Input: part model. Units: mm. Frame: model coordinates. A direction names the side the tool comes from. Round coordinates to 2 decimals unless told otherwise and drop trailing zeros. Loops run counter-clockwise (first coordinate to the right, second up) from the corner with the lowest first, then second, coordinate; pieces in that order, holes last.
(1) Access query for faces 1 (the face through (13, -732, 55)), 2 (the face through (7, -731, -62.5)). Directions: +Z, -Z, +X, -X, +Y, -Y. A direction counts if a zero-diameter tool reaches every point of the face in a straight line with its end or side. Return the directions, or none.
(2) First-contact query: pin 1 Ø3 at (y, z) = (-462.5, -25.5) entering from +X; pin 2 Ø7.5 at (y, z) = (-1442.5, -58.5) entering from -X. Flat tips, straight axial feed; report the tip coordinate or a pass-through.
(3) Cut plane B-B, the plane y = -822.5. Output: boundary loops of the cut face in (x, z).
(4) Cut plane A-A, the plane x = 11. Output: boundary loops of the cut face in (y, z).
(5) Line query: line 1 (Z direction, x = 9.5, y = -562); line 2 (Z direction, x = -14, y = -471); line 3 (X direction, y = -788, z = 49). Output: solid intervals per line, ascending.
(6) Cut plane C-C, the plane z = 23.5. Output: boundary loops of the cut face in (x, y), and give its area (3 significant figures).
(7) Draft query along Z for faces 3 (the face through (-22, -65, 23)), 4 (the face through (14, -731, -55)), 5 (the face through (8, -732, 62.5)). Return one class per face: released by +Z, released by -Z, zero draft, split by the parting line, or undercut.
from build123d import *

# Parameters (mm, degrees)
F1_DEPTH = 1482.5
F3_DEPTH = 125.001
F5_DEPTH = 10


with BuildPart() as f1:
    # F0 (on Front) → F1 (new body)
    with BuildSketch(Plane.XZ):
        with BuildLine():
            Line((-25.16784, 62.5), (-25.16784, -62.5))
            Line((-25.16784, -62.5), (39.83216, -62.5))
            Line((39.83216, -62.5), (39.83216, -55))
            Line((39.83216, -55), (-12.46784, -55))
            ThreePointArc((-12.46784, -55), (-18.124695, -52.656854), (-20.46784, -47))
            Line((-20.46784, -47), (-20.46784, 47))
            ThreePointArc((-20.46784, 47), (-18.124695, 52.656854), (-12.46784, 55))
            Line((-12.46784, 55), (39.83216, 55))
            Line((39.83216, 55), (39.83216, 62.5))
            Line((39.83216, 62.5), (-25.16784, 62.5))
        make_face()
    extrude(amount=F1_DEPTH)

    # F2 (on face) → F3 (cut, through all)
    with BuildSketch(Plane.XY.offset(62.5)):
        with BuildLine():
            Line((39.83216, 0), (-25.16784, 0))
            Line((-25.16784, 0), (-25.16784, -65))
            Line((-25.16784, -65), (-17.66784, -65))
            Line((-17.66784, -65), (-17.66784, -12.7))
            ThreePointArc((-17.66784, -12.7), (-15.324695, -7.043146), (-9.66784, -4.7))
            Line((-9.66784, -4.7), (39.83216, -4.7))
            Line((39.83216, -4.7), (39.83216, 0))
        make_face()
        with BuildLine():
            Line((-17.66784, -1417.5), (-25.16784, -1417.5))
            Line((-25.16784, -1417.5), (-25.16784, -1482.5))
            Line((-25.16784, -1482.5), (39.83216, -1482.5))
            Line((39.83216, -1482.5), (39.83216, -1477.8))
            Line((39.83216, -1477.8), (-9.66784, -1477.8))
            ThreePointArc((-9.66784, -1477.8), (-15.324695, -1475.456854), (-17.66784, -1469.8))
            Line((-17.66784, -1469.8), (-17.66784, -1417.5))
        make_face()
    extrude(amount=-F3_DEPTH, mode=Mode.SUBTRACT)

    # F4 (on face) → F5 (cut)
    with BuildSketch(Plane.XY.offset(62.5)):
        with BuildLine():
            Line((-17.66784, -65), (39.83216, -65))
            Line((39.83216, -65), (39.83216, -4.7))
            Line((39.83216, -4.7), (-9.66784, -4.7))
            ThreePointArc((-9.66784, -4.7), (-15.324695, -7.043146), (-17.66784, -12.7))
            Line((-17.66784, -12.7), (-17.66784, -65))
        make_face()
        with BuildLine():
            Line((39.83216, -1417.5), (-17.66784, -1417.5))
            Line((-17.66784, -1417.5), (-17.66784, -1469.8))
            ThreePointArc((-17.66784, -1469.8), (-15.324695, -1475.456854), (-9.66784, -1477.8))
            Line((-9.66784, -1477.8), (39.83216, -1477.8))
            Line((39.83216, -1477.8), (39.83216, -1417.5))
        make_face()
    extrude(amount=-F5_DEPTH, mode=Mode.SUBTRACT)


solid = f1.part
Reported:
1. face 1: +X, +Y, -Y
1. face 2: -Z, +X, -X, +Y, -Y
2. pin 1: stops at x = -20.47
2. pin 2: stops at x = -17.67
3. outline: (-25.17, -62.5) - (39.83, -62.5) - (39.83, -55) - (-12.47, -55) arc R8 cw to (-20.47, -47) - (-20.47, 47) arc R8 cw to (-12.47, 55) - (39.83, 55) - (39.83, 62.5) - (-25.17, 62.5) - close
4. outline: (-1477.8, -62.5) - (-4.7, -62.5) - (-4.7, -55) - (-1477.8, -55) - close; (-1417.5, 55) - (-65, 55) - (-65, 62.5) - (-1417.5, 62.5) - close
5. line 1: z = -62.5 to -55, 55 to 62.5
5. line 2: z = -62.5 to -54.85, 54.85 to 62.5
5. line 3: x = -25.17 to -20.21
6. outline: (-25.17, -1417.5) - (-20.47, -1417.5) - (-20.47, -65) - (-25.17, -65) - close
6. area: 6,360 mm2
7. face 3: zero draft
7. face 4: undercut
7. face 5: released by +Z
